Here's how the part is built. I have some questions about the finished solid (model axes, mm). Round coordinates to 2 decimals unless told otherwise and drop trailing zeros. Write each loop counter-clockwise with the first axis right and the second up, starting at its lowest first coordinate (ties: lowest second). Pieces come first, ordered by that corner, then holes. Notation, with made-up numbers: (53, 32.5) -> (57, 32.5) arc R10 ccw to (57, 45.5) -> close; hole circle Ø8 at (3, -22.75). An arc over 180 degrees is marked (long way). Answer as CSV lines item,"result".
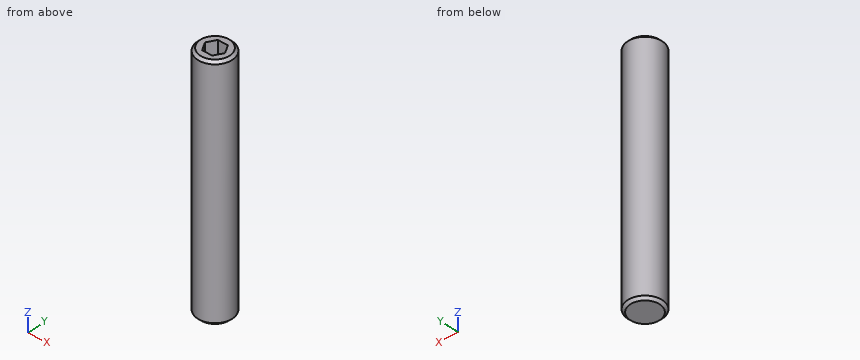
Solid Edge part; units mm, degrees
sketch "Sketch1" plane through (0, 0, 0) normal (0, 0, 1) x (1, 0, 0)
  circle A0 centre (0, 0) radius 3.175
extrude "Protrusion1" add sketch "Sketch1" along normal blind 44.45
chamfer "Chamfer1" distance 0.4762 angle 45 2 edges at (-3.175, 0, 0) (-3.175, 0, 44.45)
sketch "Sketch2" plane through (0, 0, 44.45) normal (0, 0, 1) x (1, 0, 0)
  line L0 (-0.9165, 1.5875) -> (0.9165, 1.5875)
  line L1 (1.8331, 0) -> (0.9165, 1.5875)
  line L2 (0.9165, -1.5875) -> (1.8331, 0)
  line L3 (-0.9165, -1.5875) -> (0.9165, -1.5875)
  line L4 (-1.8331, 0) -> (-0.9165, -1.5875)
  line L5 (-0.9165, 1.5875) -> (-1.8331, 0)
extrude "Cutout1" cut sketch "Sketch2" against normal blind 22.225
properties part number "162157"
1. Suppose I cut it at C-C on z = 20.5. Please give me the cut outline in (x, y) (3 decimals), and give its area (3 significant figures).
Numbers:
outline,"circle Ø6.35 at (0, 0)"
area,"31.7 mm^2"
2. For pin 1 Ø1.6 at (x, y) = (0, 0) entering from +Z (3 decimals); pin 2 Ø1 at (x, z) = (1, 15.5) entering from -Y; pin 3 Ø1.5 at (y, z) = (2, 17) entering from -X, each with a flat end and sliding along its axis, tell me the tip position at first contact or that it passes through.
Numbers:
pin 1,"stops at z = 22.225"
pin 2,"stops at y = -3.14"
pin 3,"stops at x = -2.92"
3. If I drill on line 1 (Z direction, x = -1.5, y = 0.25) (3 decimals); line 2 (Y direction, x = 1.25, z = 24.5); line 3 (Y direction, x = 0.5, z = 34), over which ranges is the centre line in solid material (lowest first)?
Numbers:
line 1,"z = 0 to 22.225"
line 2,"y = -2.92 to -1.01, 1.01 to 2.92"
line 3,"y = -3.14 to -1.59, 1.59 to 3.14"
